Could you check a few things on this drawing? It's one solid part, dimensions in mm from its lowest x, y, z. A direction names the side the tool comes from. Coordinates: 2 decimals unless noted, no trailing zeros. Loops run counter-clockwise (first coordinate to the right, second up) from the corner with the lowest first, then second, coordinate; pieces in that order, holes last. Notation, with made-up numbers: M 37.5,43 L 71.5,43 A26 cw 71.5,60 Z; hole C 85.25,-24.75 d1. An arc over 180 degrees is marked long. Use one line per item in the form item = value. Start each with the question number.
(1) Thinking about a two-plate mould opening in X: for the marked faces 3, 4 and 5, which applies, +X half, -X half, draft (parallel to the pull), parting line (faces both ways), or undercut?
(2) Imagine slicing it at A-A, the plane z = 10. Please give me the cut outline in (x, y), and give its area (3 significant figures).
(3) Will these pins go through, and if not, where does the flat tip stop? P1, Ø10, axis at x = 29.5, y = 14.5, coming from the +Z side; P2, Ø8, axis at x = 28, z = 11, coming from the +Y side; P3, Ø8, axis at x = 20, y = 5, coming from the -Z side.
(4) Imagine slicing it at C-C, the plane x = 30. Please give me the cut outline in (y, z), and give its area (3 significant figures).
(5) On a 3-axis mill with a long thin cutter (end or side, diameter ignored), from which of +Z, -Z, +X, -X, +Y, -Y can I reach the whole of each face in a straight line? I mean the marked faces 1 and 2. Say none if no direction works.
(6) Please list where these lines run through material, in increasing order: L1, parallel to X at y = 2.25, z = 7.75; L2, parallel to Y at x = 24.5, z = 10.25.
(7) Imagine slicing it at D-D, the plane z = 4. Please give me the cut outline in (x, y).
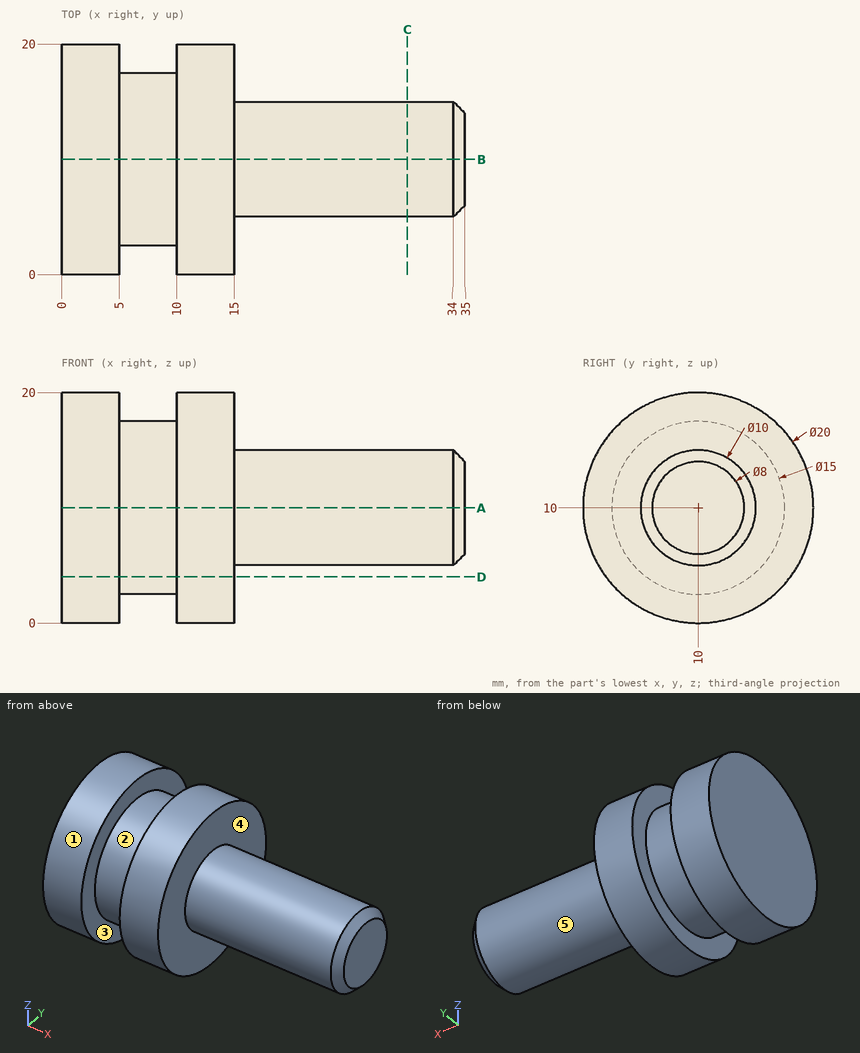
Answer:
q1.face_3 = undercut
q1.face_4 = +X half
q1.face_5 = draft
q2.outline = M 0,0 L 5,0 L 5,2.5 L 10,2.5 L 10,0 L 15,0 L 15,5 L 34,5 L 35,6 L 35,14 L 34,15 L 15,15 L 15,20 L 10,20 L 10,17.5 L 5,17.5 L 5,20 L 0,20 Z
q2.area = 474 mm²
q3.P1 = 15
q3.P2 = 15
q3.P3 = 5.1
q4.outline = C 10,10 d10
q4.area = 78.5 mm²
q5.face_1 = +X, -X
q5.face_2 = none
q6.L1 = 0 to 5, 10 to 15
q6.L2 = 5.01 to 14.99
q7.outline = M 0,2 L 5,2 L 5,5.5 L 10,5.5 L 10,2 L 15,2 L 15,18 L 10,18 L 10,14.5 L 5,14.5 L 5,18 L 0,18 Z
